The model under review builds one solid part; all positions refer to its coordinate system, in mm. A direction names the side the tool comes from. Coordinates: 2 decimals unless noted, no trailing zeros. Order: outer loops, then holes, each group sorted by start corner. A loop starts at its lowest first (then second) coordinate and runs counter-clockwise, first axis right, second up.
```python
from build123d import *

# Parameters (mm, degrees)
CUT_EXTRUDE1_DEPTH = 1.5


with BuildPart() as part:
    # Sketch1 → Revolve1 (revolve)
    with BuildSketch(Plane.XY):
        Polygon((0, 0), (25, 0), (25, 2), (20, 2), (20, 2.5), (4, 2.5), (4, 4), (0, 4), align=None)
    revolve(axis=Axis((0, 0, 0), (1, 0, 0)))

    # Sketch2 → Cut-Extrude1 (cut)
    with BuildSketch(Plane.ZY):
        Polygon((-0.209897737, 1.428032308), (-1.341661125, 0.532239381), (-1.131763388, -0.895792927), (0.209897737, -1.428032308), (1.341661125, -0.532239381), (1.131763388, 0.895792927), align=None)
    extrude(amount=-CUT_EXTRUDE1_DEPTH, mode=Mode.SUBTRACT)


solid = part.part
```
(1) Machinability: for faces 1 (the face through (22, 0, -2)), 2 (the face through (0, -1, 1)), 3 (the face through (0.74, 1.16, 0.47)), which of the approach directions +Z, -Z, +X, -X, +Y, -Y give a long, thin tool a straight path to every point of the face, cutting with its end or side? Answer none if there is none.
A:
face 1: +X
face 2: +Z, -Z, -X, +Y, -Y
face 3: -X
(2) For pin 1 Ø1.5 at (y, z) = (0.5, 0.5) entering from -X; pin 2 Ø3 at (x, y) = (15.5, -1.5) entering from -Z; pin 3 Ø4 at (x, z) = (10, 2) entering from -Y; pin 4 Ø1.5 at (x, z) = (5, -0.5) entering from +Y, all flat-tipped, find the tip position at first contact; note any pin that passes through.
A:
pin 1: stops at x = 0
pin 2: stops at z = -2.5
pin 3: stops at y = -2.5
pin 4: stops at y = 2.5
(3) We need section B-B, the plane y = 0. Write out the cut boundary in (x, z).
A:
outline: (0, -4) - (4, -4) - (4, -2.5) - (20, -2.5) - (20, -2) - (25, -2) - (25, 2) - (20, 2) - (20, 2.5) - (4, 2.5) - (4, 4) - (0, 4) - (0, 1.26) - (1.5, 1.26) - (1.5, -1.26) - (0, -1.26) - close
(4) We need section C-C, the plane x = 14. Write out the cut boundary in (y, z).
A:
outline: circle Ø5 at (0, 0)
(5) We need section A-A, the plane z = -1.75. Write out the cut boundary in (x, y).
A:
outline: (0, -3.6) - (4, -3.6) - (4, -1.79) - (20, -1.79) - (20, -0.97) - (25, -0.97) - (25, 0.97) - (20, 0.97) - (20, 1.79) - (4, 1.79) - (4, 3.6) - (0, 3.6) - close
(6) We need section D-D, the plane y = 3.5. Write out the cut boundary in (x, z), and give its area (3 significant figures).
A:
outline: (0, -1.94) - (4, -1.94) - (4, 1.94) - (0, 1.94) - close
area: 15.5 mm2
(7) Wall thickness on probe 1 along Y at (x, z) = (12.75, -1.5); probe 2 along X at (y, z) = (2.75, 0.25); probe 3 along Z at (x, y) = (16.5, 0.25): over which ranges is each line inside the solid? List them lowest first.
A:
probe 1: y = -2 to 2
probe 2: x = 0 to 4
probe 3: z = -2.49 to 2.49
(8) Draft analysis for pull direction Y (two halves, no side actions). For faces 4 (the face through (25, 0, 0)), 5 (the face through (11.89, -0.54, -2.44)), 6 (the face through (0.74, -1.16, -0.47)), state which applies: released by +Y, released by -Y, zero draft, split by the parting line, or undercut.
A:
face 4: zero draft
face 5: split by the parting line
face 6: undercut
